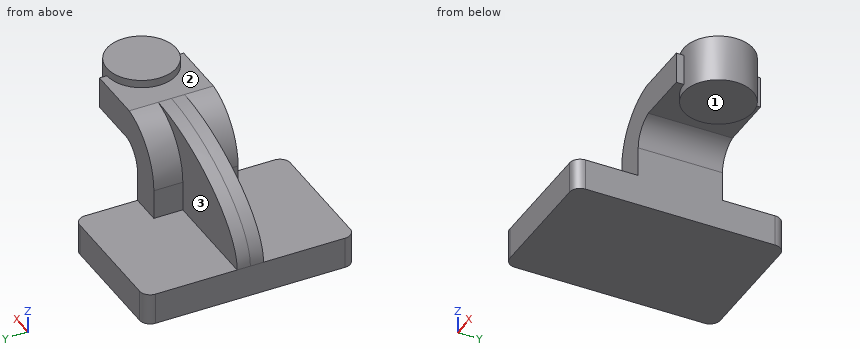
from build123d import *

# Parameters (mm, degrees)
F1_DEPTH = 63.5
F0_W     = 29.9330746515
F0_H     = 19.05
F2_DEPTH = 25.4
F3_DEPTH = 7.9375
F5_R     = 6.35


# Not quite as in the source:
# - the program builds the solid bodies; features that only make, move or delete a surface that nothing else refers to are left out


with BuildPart() as f1:
    # F0 (on Front) → F1 (new body, symmetric)
    with BuildSketch(Plane.XZ):
        Polygon((-41.275, 9.525), (-41.275, -9.525), (41.275, -9.525), (41.275, 9.525), (22.225, 9.525), align=None)
    extrude(amount=F1_DEPTH, both=True)

    # F0 (on Front) → F2 (join, symmetric)
    with BuildSketch(Plane.XZ):
        with BuildLine():
            Line((22.225, 9.525), (41.275, 9.525))
            Line((41.275, 9.525), (41.275, 27.5486753512))
            ThreePointArc((41.275, 27.5486753512), (44.5496824671, 37.2051562356), (53.0227320404, 42.8777746134))
            Line((53.0227320404, 42.8777746134), (55.8209344745, 42.8777746134))
            Line((55.8209344745, 42.8777746134), (55.8209344745, 61.9277746134))
            Line((55.8209344745, 61.9277746134), (50.9991334821, 61.9277746134))
            ThreePointArc((50.9991334821, 61.9277746134), (30.3677797958, 49.9644801757), (22.225, 27.5486753512))
            Line((22.225, 27.5486753512), (22.225, 9.525))
        make_face()
        with Locations((70.7874718002, 52.4027746134)):
            Rectangle(F0_W, F0_H)
    extrude(amount=F2_DEPTH, both=True)

    # F0 (on Front) → F3 (join, symmetric)
    with BuildSketch(Plane.XZ):
        with BuildLine():
            add(Edge.make_bspline(
                [(-41.275, 9.525), (-41.3442589343, 36.1172966659), (8.2413451746, 61.5874938667), (50.9991334821, 61.9277746134)],
                knots=[0, 0, 0, 0, 106.1158164321, 106.1158164321, 106.1158164321, 106.1158164321], degree=3))
            Line((-41.275, 9.525), (22.225, 9.525))
            Line((22.225, 9.525), (22.225, 27.5486753512))
            ThreePointArc((22.225, 27.5486753512), (30.3677797958, 49.9644801757), (50.9991334821, 61.9277746134))
        make_face()
    extrude(amount=F3_DEPTH, both=True)

    # F0 (on Front) → F4 (revolve)
    with BuildSketch(Plane.XZ):
        Polygon((85.754009126, 66.675), (85.754009126, 61.9277746134), (85.754009126, 42.8777746134), (85.754009126, 38.1), (106.6209344745, 38.1), (106.6209344745, 66.675), align=None)
    revolve(axis=Axis((85.754009126, 0, 52.3875), (0, 0, -1)))

    # F5
    f5_edges = [f1.edges().sort_by_distance(p)[0] for p in [
        (-41.275, -63.5, 0),
        (41.275, -63.5, 0),
        (-41.275, 63.5, 0),
        (41.275, 63.5, 0),
    ]]
    fillet(f5_edges, radius=F5_R)


solid = f1.part
Design review of the part built by this model. Coordinates are the model's own, in mm. Face numbers are marked on the shaded views. A direction names the side the tool comes from. Round coordinates to 2 decimals unless told otherwise and drop trailing zeros. Loops run counter-clockwise (first coordinate to the right, second up) from the corner with the lowest first, then second, coordinate; pieces in that order, holes last. Notation, with made-up numbers: M 44.5,-15 L 68.5,-15 A11 ccw 68.5,-5 Z; hole C 48,-19.75 d4. An arc over 180 degrees is marked long. Answer as a JSON object with one key per item and string values.
Item 1: Wall thickness on L1, parallel to Z at x = -17, y = 17 (3 decimals); L2, parallel to Y at x = 4.5, z = 10.5; L3, parallel to Y at x = 69, z = 58: over which ranges is each line inside the solid? List them lowest first. Write a range as from..to.
Answer sheet:
{"L1": "z = -9.525..9.525", "L2": "y = -7.94..7.94", "L3": "y = -25.4..25.4"}
Item 2: Machinability: for the marked faces 1, 2 and 3, which of the approach directions +Z, -Z, +X, -X, +Y, -Y give a long, thin tool a straight path to every point of the face, cutting with its end or side? Answer none if there is none.
Answer sheet:
{"face 1": "-Z, +X, +Y, -Y", "face 2": "+Z, -X", "face 3": "+Z, -X, +Y"}
Item 3: We need section B-B on y = 45.5. Give the boundary of the cut face in (x, z) (3 decimals).
Answer sheet:
{"outline": "M -41.275,-9.525 L 41.275,-9.525 L 41.275,9.525 L -41.275,9.525 Z"}
Item 4: We need section C-C on y = 11.5. Give the boundary of the cut face in (x, z) (3 decimals).
Answer sheet:
{"outline": "M -41.275,-9.525 L 41.275,-9.525 L 41.275,27.549 A15.875 cw 53.023,42.878 L 68.342,42.878 L 68.342,38.1 L 103.166,38.1 L 103.166,66.675 L 68.342,66.675 L 68.342,61.928 L 50.999,61.928 A34.925 ccw 22.225,27.549 L 22.225,9.525 L -41.275,9.525 Z"}
Item 5: We need section A-A on y = -18. Give the boundary of the cut face in (x, z) (3 decimals), and give its area (3 significant figures).
Answer sheet:
{"outline": "M -41.275,-9.525 L 41.275,-9.525 L 41.275,27.549 A15.875 cw 53.023,42.878 L 75.198,42.878 L 75.198,38.1 L 96.31,38.1 L 96.31,66.675 L 75.198,66.675 L 75.198,61.928 L 50.999,61.928 A34.925 ccw 22.225,27.549 L 22.225,9.525 L -41.275,9.525 Z", "area": "3,620 mm^2"}
Item 6: Clearance check with flat-ended pins moving along their axes: P1, Ø4, axis at x = -6, y = 28.5, coming from the +Z side (3 decimals); P2, Ø11, axis at y = -20, z = 5, coming from the +X side (3 decimals); P3, Ø5, axis at y = 15.5, z = 18, coming from the -X side (3 decimals); P4, Ø12, axis at x = 48, z = 13.5, coming from the +Y side. State where each tip first meets the part, or that it passes through.
Answer sheet:
{"P1": "stops at z = 9.525", "P2": "stops at x = 41.275", "P3": "stops at x = 22.225", "P4": "passes through"}
